Could you check a few things on this drawing? It's one solid part, dimensions in mm from its lowest x, y, z. A direction names the side the tool comes from. Give positions to 0.01 mm unless a question says otherwise; leave off trailing zeros. Loops run counter-clockwise (first coordinate to the right, second up) from the corner with the lowest first, then second, coordinate; pieces in that order, holes last. Notation, with made-up numbers: M 19,-9 L 54,-9 A22 ccw 54,30 Z; hole C 83,-5.5 d7. An arc over 180 degrees is marked long. Answer in a Markdown table with one row per item. Add a question column.
1. I'm going to push flat-ended pins straight in: pin 1 Ø4 at (y, z) = (7.5, 39) entering from +X; pin 2 Ø1.5 at (x, y) = (16.5, 38.5) entering from -Z; pin 3 Ø8 at (x, z) = (30, 16.5) entering from +Y; pin 4 Ø1.5 at (x, z) = (49.5, 17) entering from +Y (1 decimal). Where does each tip first touch, or does it pass through?
2. Which directions (+Z, -Z, +X, -X, +Y, -Y) give clear straight access to the entire face, cutting with the end or side of a thin tool? Please do the marked faces 1, 2 and 3.
3. If we section it at A-A on z = 31: List the corners of the cut face in (x, y) for me (1 decimal).
4. I need wall thicknesses on line 1 along Z through (x, y) = (22.5, 20); line 2 along Z through (x, y) = (46, 9) (1 decimal); line 3 along Y through (x, z) = (44, 22.5) (1 decimal). Which ranges of each line are inside material? Lowest first, please. Write a range as from..to.
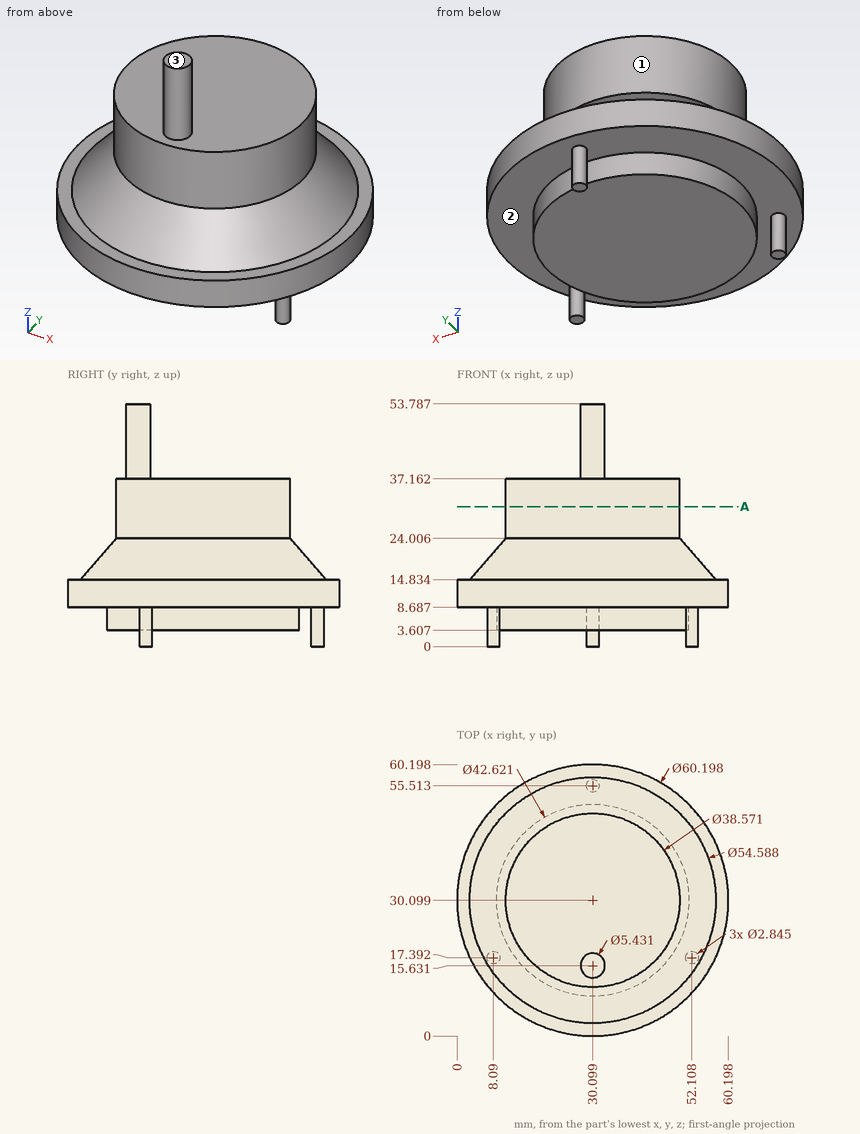
Results:
| question | item | result |
|---|---|---|
| 1 | pin 1 | through |
| 1 | pin 2 | z = 3.61 |
| 1 | pin 3 | y = 60.2 |
| 1 | pin 4 | y = 47.8 |
| 2 | face 1 | +Z |
| 2 | face 2 | -Z |
| 2 | face 3 | +Z, +X, -X, +Y, -Y |
| 3 | outline | C 30.1,30.1 d38.6 |
| 4 | line 1 | 3.61..37.16 |
| 4 | line 2 | 8.7..15.8 |
| 4 | line 3 | 14.9..45.3 |
